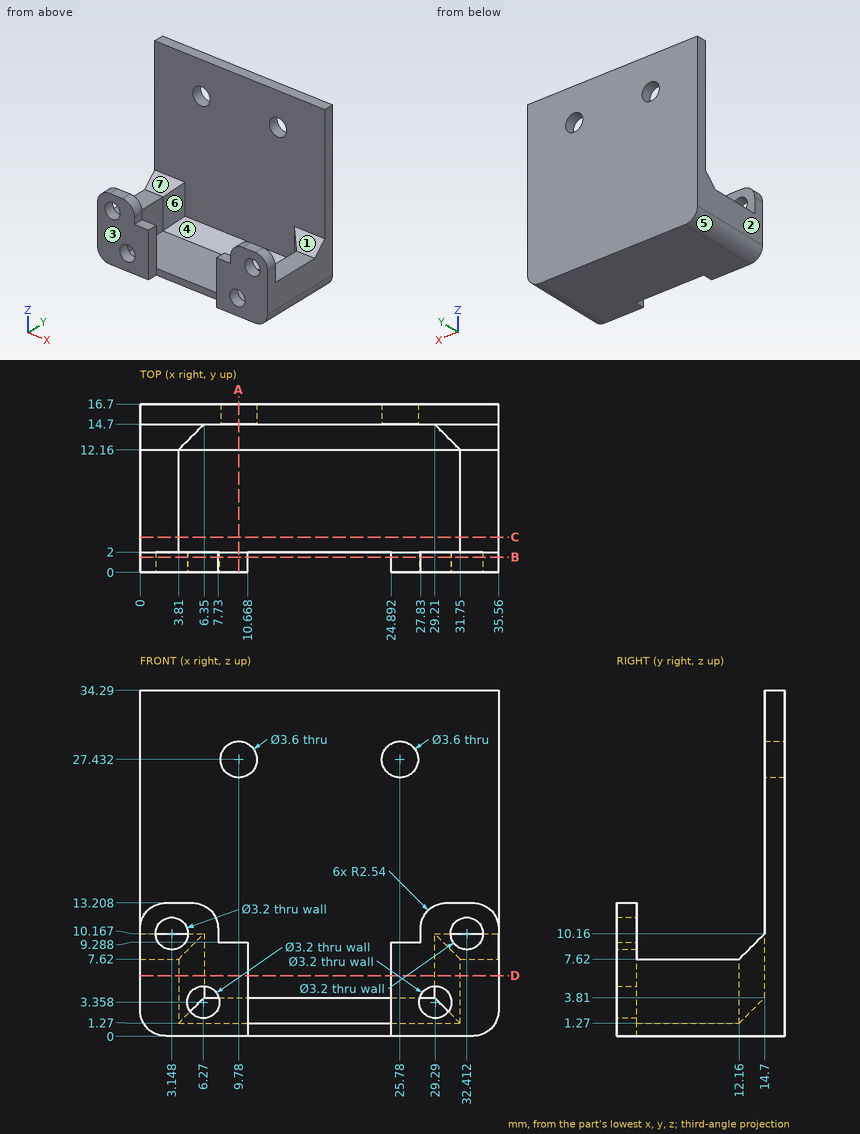
The figure shows three views and two pictorial views of one solid part (mm, origin at its lowest corner). Answer the questions. A direction names the side the tool comes from. Give positions to 0.01 mm unless a question says otherwise; leave off trailing zeros. Order: outer loops, then holes, each group sorted by start corner. A loop starts at its lowest first (then second) coordinate and runs counter-clockwise, first axis right, second up. Notation, with made-up numbers: (29.5, -34) -> (88.5, -34) arc R12 cw to (88.5, -19) -> close; hole circle Ø3 at (-31, 86.25). An arc over 180 degrees is marked (long way). One line per item, written item: value.
1) A tool of negligible diameter and unlimited length cuts with its end or side. For the marked faces 5, 6 and 7, from which of +Z, -Z, +X, -X, +Y, -Y can it reach the whole face along a straight path? Write none if from no direction.
Reported:
face 5: -Z, -X, +Y, -Y
face 6: +Z
face 7: +Z, +X, -X
2) Find section B-B, the plane y = 1.5. Determine the outline of the cut face in (x, z).
Reported:
outline: (0, 2.54) arc R2.54 ccw to (2.54, 0) -> (10.67, 0) -> (10.67, 9.29) -> (7.73, 9.29) -> (7.73, 10.67) arc R2.54 ccw to (5.19, 13.21) -> (2.54, 13.21) arc R2.54 ccw to (0, 10.67) -> close; (24.89, 0) -> (33.02, 0) arc R2.54 ccw to (35.56, 2.54) -> (35.56, 10.67) arc R2.54 ccw to (33.02, 13.21) -> (30.37, 13.21) arc R2.54 ccw to (27.83, 10.67) -> (27.83, 9.29) -> (24.89, 9.29) -> close; hole circle Ø3.2 at (3.15, 10.17); hole circle Ø3.2 at (6.27, 3.36); hole circle Ø3.2 at (29.29, 3.36); hole circle Ø3.2 at (32.41, 10.17)
3) Find the intervals of material crossed by line 1 (X direction, y = 9, z = 3.5); line 2 (Y direction, x = 34.5, z = 29.5); line 3 (Z direction, x = 8, y = 5.75), in increasing order.
Reported:
line 1: x = 0 to 3.81, 31.75 to 35.56
line 2: y = 14.7 to 16.7
line 3: z = 0 to 1.27
4) Find section D-D, the plane z = 6. Determine the outline of the cut face in (x, y).
Reported:
outline: (0, 0) -> (10.67, 0) -> (10.67, 2) -> (3.81, 2) -> (3.81, 12.16) -> (6.35, 14.7) -> (29.21, 14.7) -> (31.75, 12.16) -> (31.75, 2) -> (24.89, 2) -> (24.89, 0) -> (35.56, 0) -> (35.56, 16.7) -> (0, 16.7) -> close
5) Flat-ended cylindrical pins translate along their axes: P1, Ø8, axis at x = 22, y = 8.5, coming from the +Z side; P2, Ø6, axis at x = 13.5, y = 6, coming from the +Z side; P3, Ø2, axis at x = 9.78, z = 27.432, coming from the -Y side; P4, Ø8, axis at x = 28.5, z = 23.5, coming from the -Y side. Find the tip coordinate at first contact, or state that the pin passes through.
Reported:
P1: stops at z = 1.61
P2: stops at z = 1.27
P3: passes through
P4: stops at y = 14.7
6) Determine the mould class of the marked faces 1, 2, 3 and 4 for opening direction Y: pulls with the +Y half, pulls with the -Y half, needs draft (parallel to the pull), parting line crosses it, or undercut.
Reported:
face 1: undercut
face 2: needs draft
face 3: pulls with the -Y half
face 4: undercut
7) Find section A-A, the plane x = 9.78. Determine the outline of the cut face in (y, z).
Reported:
outline: (0, 0) -> (16.7, 0) -> (16.7, 25.63) -> (14.7, 25.63) -> (14.7, 3.81) -> (12.16, 1.27) -> (2, 1.27) -> (2, 9.29) -> (0, 9.29) -> close; (14.7, 29.23) -> (16.7, 29.23) -> (16.7, 34.29) -> (14.7, 34.29) -> close
8) Find section C-C, the plane y = 3.5. Determine the outline of the cut face in (x, z).
Reported:
outline: (0, 2.54) arc R2.54 ccw to (2.54, 0) -> (33.02, 0) arc R2.54 ccw to (35.56, 2.54) -> (35.56, 7.62) -> (31.75, 7.62) -> (31.75, 1.27) -> (3.81, 1.27) -> (3.81, 7.62) -> (0, 7.62) -> close
